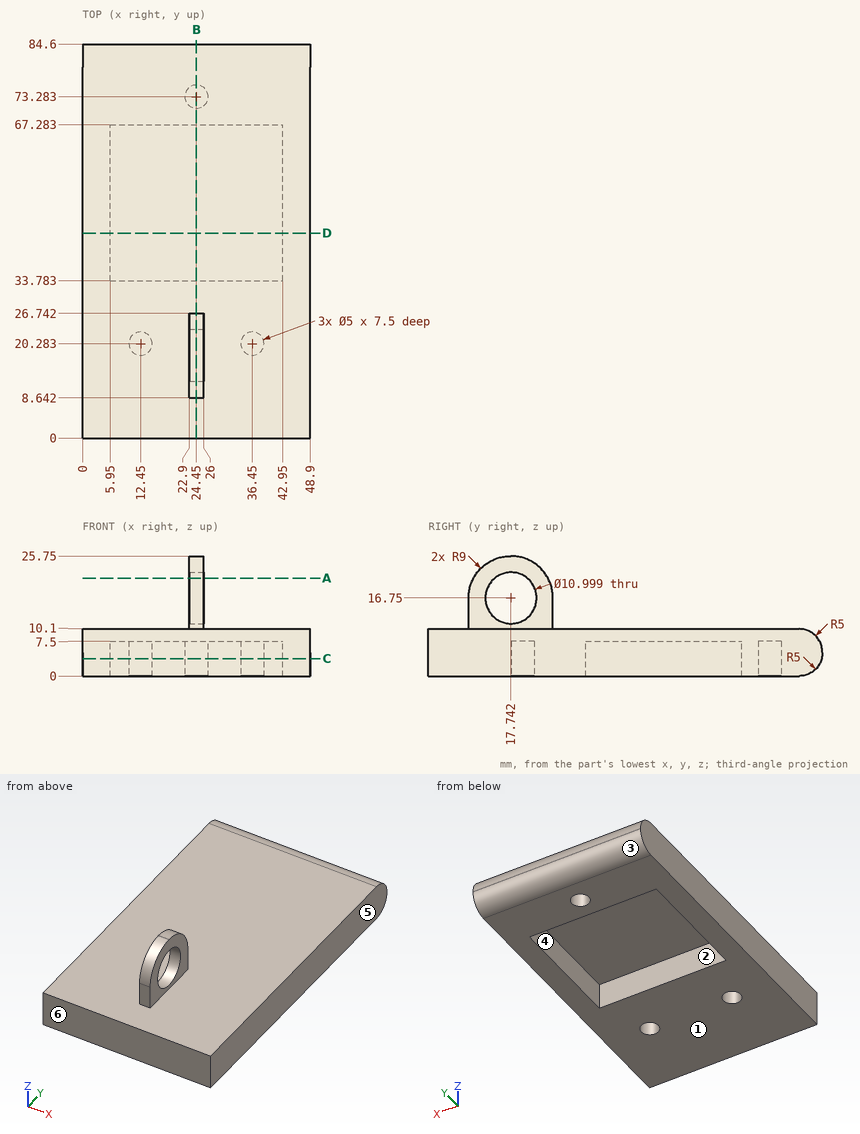
Geometry check sheet. Reference: drawing and pictorial views, mm from the part's lowest x, y, z. A direction names the side the tool comes from. Round coordinates to 2 decimals unless told otherwise and drop trailing zeros. Write each loop counter-clockwise with the first axis right and the second up, starting at its lowest first coordinate (ties: lowest second). Pieces come first, ordered by that corner, then holes.
(1) Section check A-A (z = 21). Enter the section's corners in (x, y) (1 decimal).
Returned:
outline: (22.9, 9.7) - (26, 9.7) - (26, 14.3) - (22.9, 14.3) - close; (22.9, 21.2) - (26, 21.2) - (26, 25.7) - (22.9, 25.7) - close
(2) Material ranges on line 1 (Y direction, x = 12.45, z = 5.25); line 2 (Y direction, x = 31.5, z = 5.5); line 3 (Y direction, x = 12.45, z = 2.25) (1 decimal), recorded low to high.
Returned:
line 1: y = 0 to 17.78, 22.78 to 33.78, 67.28 to 84.6
line 2: y = 0 to 33.78, 67.28 to 84.58
line 3: y = 0 to 17.8, 22.8 to 33.8, 67.3 to 83.8
(3) Mould release check, pull along Y, two halves, no side actions. Record for the marked faces 3, 4, 5 and 6: pulls with the +Y half, pulls with the -Y half, needs draft (parallel to the pull), parting line crosses it, or undercut.
Returned:
face 3: pulls with the +Y half
face 4: undercut
face 5: needs draft
face 6: pulls with the -Y half
(4) Section check C-C (z = 3.75). Enter the section's corners in (x, y).
Returned:
outline: (0, 0) - (48.9, 0) - (48.9, 84.44) - (0, 84.44) - close; hole (5.95, 33.78) - (42.95, 33.78) - (42.95, 67.28) - (5.95, 67.28) - close; hole circle Ø5 at (12.45, 20.28); hole circle Ø5 at (24.45, 73.28); hole circle Ø5 at (36.45, 20.28)
(5) Depth check by flat-ended pin: pin 1 Ø8 at (x, y) = (22, 11) entering from +Z; pin 2 Ø10 at (y, z) = (17.74, 16.75) entering from +X; pin 3 Ø3 at (x, y) = (24.45, 73.28) entering from -Z; pin 4 Ø4 at (x, y) = (12.45, 20.28) entering from +Z. Enter the tip coordinate at first touch or a pass-through.
Returned:
pin 1: stops at z = 25.32
pin 2: passes through
pin 3: stops at z = 7.5
pin 4: stops at z = 10.1
(6) Section check B-B (x = 24.45). Enter the section's corners in (y, z).
Returned:
outline: (0, 0) - (33.78, 0) - (33.78, 7.5) - (67.28, 7.5) - (67.28, 0) - (70.78, 0) - (70.78, 7.5) - (75.78, 7.5) - (75.78, 0) - (79.6, 0) arc R5 ccw to (84.6, 5) - (84.6, 5.1) arc R5 ccw to (79.6, 10.1) - (26.74, 10.1) - (26.74, 16.75) arc R9 ccw to (17.74, 25.75) - (17.64, 25.75) arc R9 ccw to (8.64, 16.75) - (8.64, 10.1) - (0, 10.1) - close; hole circle Ø11 at (17.74, 16.75)
(7) Section check D-D (y = 44). Enter the section's corners in (x, z), plus the area to 3 significant figures.
Returned:
outline: (0, 0) - (5.95, 0) - (5.95, 7.5) - (42.95, 7.5) - (42.95, 0) - (48.9, 0) - (48.9, 10.1) - (0, 10.1) - close
area: 216 mm2
(8) Access from +Z, -Z, +X, -X, +Y, -Y to the whole of each face (thin tool, end or side, straight path). Record for the marked faces 1 and 2.
Returned:
face 1: -Z, +X, -X, +Y, -Y
face 2: -Z
